from build123d import *

# Parameters (mm, degrees)
SKETCH_R     = 2
PAD_DEPTH    = 3
PAD001_DEPTH = 27


with BuildPart() as part:
    # Sketch → Pad (new body)
    with BuildSketch(Plane.XY):
        with BuildLine():
            ThreePointArc((100.142058, 282.792447), (0, 300), (-100.142058, 282.792447))
            Line((-100.142058, 282.792447), (-99.140637, 279.964523))
            ThreePointArc((-35, 294.9305), (-67.486464, 289.23101), (-99.140637, 279.964523))
            Line((-35, 294.9305), (-30, 275))
            Line((-30, 275), (30, 275))
            Line((30, 275), (35, 294.9305))
            ThreePointArc((99.140637, 279.964523), (67.486464, 289.23101), (35, 294.9305))
            Line((100.142058, 282.792447), (99.140637, 279.964523))
        make_face()
        with Locations((-17.5, 285)):
            Circle(SKETCH_R, mode=Mode.SUBTRACT)
        with Locations((17.5, 285)):
            Circle(SKETCH_R, mode=Mode.SUBTRACT)
    extrude(amount=PAD_DEPTH)

    # Sketch001 (on Face12 of Pad) → Pad001 (join)
    with BuildSketch(Plane.XY.offset(3)):
        with BuildLine():
            ThreePointArc((100.142058, 282.792447), (0, 300), (-100.142058, 282.792447))
            Line((-100.142058, 282.792447), (-99.140637, 279.964523))
            ThreePointArc((99.140637, 279.964523), (0, 297), (-99.140637, 279.964523))
            Line((100.142058, 282.792447), (99.140637, 279.964523))
        make_face()
    extrude(amount=PAD001_DEPTH)


solid = part.part
Geometry check sheet. Reference: the model listing, model coordinates, mm. A direction names the side the tool comes from. Round coordinates to 2 decimals unless told otherwise and drop trailing zeros. Order: outer loops, then holes, each group sorted by start corner. A loop starts at its lowest first (then second) coordinate and runs counter-clockwise, first axis right, second up. Notation, with made-up numbers: M -16.75,76.25 L 32.25,76.25 A26 ccw 32.25,95.25 Z; hole C 78,12 d4. An arc over 180 degrees is marked long. Answer in a Markdown table with one row per item. Add a question column.
Item 1: Material ranges on L1, parallel to Z at x = 3, y = 281.5; L2, parallel to Y at x = 17.5, z = 0.9; L3, parallel to Y at x = 28.5, z = 2, recorded low to high. Write a range as [from, to].
Item 2: Sectioned sample at B-B, the plane x = 17.5. Enter the section's corners in (y, z), plus the area to 3 significant figures.
Item 3: Sectioned sample at A-A, the plane y = 285. Enter the section's corners in (x, z), plus the area to 3 significant figures.
Item 4: Set-up check for faces 4 (the face through (-67.036, 289.336, 1.479)), 5 (the face through (-0.5, 297.4, 30)), 6 (the face through (1, 297, 16)): record each of +Z, -Z, +X, -X, +Y, -Y from which the full face is reachable in a straight line by a thin tool's end or side.
Item 5: Depth check by flat-ended pin: pin 1 Ø1.5 at (x, y) = (-17.5, 279) entering from -Z; pin 2 Ø5 at (x, y) = (17.5, 285) entering from +Z; pin 3 Ø1.5 at (y, z) = (279.5, 7.5) entering from +X; pin 4 Ø10 at (y, z) = (287.5, 5) entering from -X. Enter the tip coordinate at first touch or a pass-through.
Item 6: Draft check along X on faces 1 (the face through (-1, 288, 0)), 2 (the face through (1, 300, 15)), 3 (the face through (67.936, 289.126, 1.479)). Enter one of: released by +X, released by -X, zero draft, split by the parting line, or undercut.
Item 7: Sectioned sample at D-D, the plane y = 277. Enter the section's corners in (x, z), plus the area to 3 significant figures.
Item 8: Sectioned sample at C-C, the plane y = 292.5. Enter the section's corners in (x, z), plus the area to 3 significant figures.
Filled in:
| question | item | result |
|---|---|---|
| 1 | L1 | z = [0, 3] |
| 1 | L2 | y = [275, 283], [287, 299.49] |
| 1 | L3 | y = [275, 298.64] |
| 2 | outline | M 275,0 L 283,0 L 283,3 L 275,3 Z; M 287,0 L 299.49,0 L 299.49,30 L 296.48,30 L 296.48,3 L 287,3 Z |
| 2 | area | 143 mm² |
| 3 | outline | M -93.67,0 L -83.57,0 L -83.57,30 L -93.67,30 Z; M -32.51,0 L -19.5,0 L -19.5,3 L -32.51,3 Z; M -15.5,0 L 15.5,0 L 15.5,3 L -15.5,3 Z; M 19.5,0 L 32.51,0 L 32.51,3 L 19.5,3 Z; M 83.57,0 L 93.67,0 L 93.67,30 L 83.57,30 Z |
| 3 | area | 777 mm² |
| 4 | face 4 | +Z, -Z, -Y |
| 4 | face 5 | +Z, +X, -X, +Y, -Y |
| 4 | face 6 | +Z, -Y |
| 5 | pin 1 | stops at z = 0 |
| 5 | pin 2 | stops at z = 3 |
| 5 | pin 3 | stops at x = 99.24 |
| 5 | pin 4 | stops at x = -100.14 |
| 6 | face 1 | zero draft |
| 6 | face 2 | split by the parting line |
| 6 | face 3 | undercut |
| 7 | outline | M -30.5,0 L 30.5,0 L 30.5,3 L -30.5,3 Z |
| 7 | area | 183 mm² |
| 8 | outline | M -66.66,0 L -51.5,0 L -51.5,30 L -66.66,30 Z; M -34.39,0 L 34.39,0 L 34.39,3 L -34.39,3 Z; M 51.5,0 L 66.66,0 L 66.66,30 L 51.5,30 Z |
| 8 | area | 1,120 mm² |
